For this review, take the finished solid that the model builds, in its own axes (mm). Give positions to 0.01 mm unless a question says otherwise; leave off trailing zeros. Order: outer loops, then holes, each group sorted by start corner. A loop starts at its lowest first (then second) coordinate and runs counter-clockwise, first axis right, second up. Notation, with made-up numbers: (4, 13) - (38, 13) arc R21 ccw to (38, 46) - close; hole circle Ø9 at (55, 63.5). An arc over 180 degrees is marked (long way). Use a Markdown table: item, result. Add a question column.
1) We need section B-B on y = 39.5. Write out the cut boundary in (x, z).
2) Clearance check with flat-ended pins moving along their axes: P1, Ø0.9, axis at y = 72.5, z = 1.5, coming from the -X side; P2, Ø1.5, axis at x = 4, z = 1.5, coming from the +Y side; P3, Ø3, axis at x = 99, y = 101, coming from the -Z side; P4, Ø1.5, axis at y = 55, z = 2, coming from the -X side. State where each tip first meets the part, or that it passes through.
3) Wall thickness on L1, parallel to X at y = 122.5, z = 1.4; L2, parallel to X at y = 70, z = 1.85; L3, parallel to Y at x = 13.5, z = 2.1: over which ranges is each line inside the solid? List them lowest first.
4) We need section A-A on z = 1.7. Write out the cut boundary in (x, y), then the cut area to 3 significant figures.
```python
from build123d import *

# Parameters (mm, degrees)
EXTRUDE_1_DEPTH = 3
FILLET_1_R      = 0.5
FILLET_2_R      = 1


with BuildPart() as part:
    # Model → 凸台-拉伸1 (new body)
    with BuildSketch(Plane.XY):
        Polygon((204.883, 129.021), (6.45693, 129.021), (6.45693, 108.371), (1.69393, 108.371), (1.69393, 82.991), (11.21893, 82.991), (11.21893, 63.941), (15.98193, 63.941), (15.98193, 44.891), (25.50693, 44.891), (25.50693, 22.641), (15.98193, 22.641), (15.98193, 0.434082), (204.883, 0.434082), align=None)
    extrude(amount=EXTRUDE_1_DEPTH)

    # 圆角1
    fillet_1_edges = [part.edges().sort_by_distance(p)[0] for p in [
        (15.98193, 22.641, 1.5),
        (25.50693, 22.641, 1.5),
        (25.50693, 44.891, 1.5),
        (15.98193, 44.891, 1.5),
        (15.98193, 63.941, 1.5),
        (11.21893, 63.941, 1.5),
        (11.21893, 82.991, 1.5),
        (1.69393, 82.991, 1.5),
        (1.69393, 108.371, 1.5),
        (6.45693, 108.371, 1.5),
    ]]
    fillet(fillet_1_edges, radius=FILLET_1_R)

    # 圆角2
    fillet_2_edges = [part.edges().sort_by_distance(p)[0] for p in [
        (6.45693, 129.021, 1.5),
        (204.883, 129.021, 1.5),
        (204.883, 0.434082, 1.5),
        (15.98193, 0.434082, 1.5),
    ]]
    fillet(fillet_2_edges, radius=FILLET_2_R)


solid = part.part
```
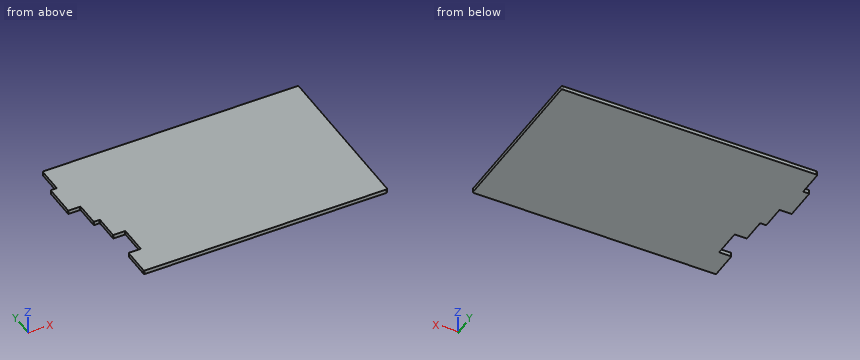
Checked values:
| question | item | result |
|---|---|---|
| 1 | outline | (25.51, 0) - (204.88, 0) - (204.88, 3) - (25.51, 3) - close |
| 2 | P1 | x = 11.22 |
| 2 | P2 | y = 108.37 |
| 2 | P3 | z = 0 |
| 2 | P4 | x = 15.98 |
| 3 | L1 | 6.46 to 204.88 |
| 3 | L2 | 11.22 to 204.88 |
| 3 | L3 | 63.94 to 129.02 |
| 4 | outline | (1.69, 83.49) arc R0.5 ccw to (2.19, 82.99) - (10.72, 82.99) arc R0.5 cw to (11.22, 82.49) - (11.22, 64.44) arc R0.5 ccw to (11.72, 63.94) - (15.48, 63.94) arc R0.5 cw to (15.98, 63.44) - (15.98, 45.39) arc R0.5 ccw to (16.48, 44.89) - (25.01, 44.89) arc R0.5 cw to (25.51, 44.39) - (25.51, 23.14) arc R0.5 cw to (25.01, 22.64) - (16.48, 22.64) arc R0.5 ccw to (15.98, 22.14) - (15.98, 1.43) arc R1 ccw to (16.98, 0.43) - (203.88, 0.43) arc R1 ccw to (204.88, 1.43) - (204.88, 128.02) arc R1 ccw to (203.88, 129.02) - (7.46, 129.02) arc R1 ccw to (6.46, 128.02) - (6.46, 108.87) arc R0.5 cw to (5.96, 108.37) - (2.19, 108.37) arc R0.5 ccw to (1.69, 107.87) - close |
| 4 | area | 24,700 mm² |
